The model under review builds one solid part; all positions refer to its coordinate system, in mm. Face numbers are marked on the shaded views. A direction names the side the tool comes from. Coordinates: 2 decimals unless noted, no trailing zeros. Loops run counter-clockwise (first coordinate to the right, second up) from the corner with the lowest first, then second, coordinate; pieces in that order, holes last. Notation, with made-up numbers: M 70,36.25 L 117,36.25 A23 cw 117,52.25 Z; hole C -11,28.25 d7. An arc over 180 degrees is marked long. Write item = value, one per line. Start each with the question number.
Q1. Mouldability with a two-part tool opening along Y and no side actions: class the marked faces 4, 5, 6 and 7 as released by +Y, released by -Y, zero draft, split by the parting line, or undercut.
Q2. Clearance check with flat-ended pins moving along their axes: pin 1 Ø0.8 at (x, z) = (-12.5, 3) entering from -Y; pin 2 Ø1.5 at (y, z) = (7.5, 2.5) entering from -X; pin 3 Ø6 at (x, z) = (-7, 1.5) entering from -Y. State where each tip first meets the part, or that it passes through.
Q3. We need section C-C on z = 9. Give the boundary of the cut face in (x, y), and give its area (3 significant figures).
Q4. For the marked faces 1, 2 and 3, list the 3-axis set-ups (+Z, -Z, +X, -X, +Y, -Y) from which the entire face can be reached by the end or side of a thin tool; tool diameter is ignored.
Q5. We need section B-B on x = 2.5. Give the boundary of the cut face in (y, z), and give its area (3 significant figures).
Q6. We need section D-D on x = -6.5. Give the boundary of the cut face in (y, z).
Q7. Wall thickness on probe 1 along X at (y, z) = (0.25, 1.25); probe 2 along Y at (x, z) = (-1, 9); probe 3 along Y at (x, z) = (4.25, 6.75): over which ranges is each line inside the solid? List them lowest first.
Q8. We need section A-A on y = 1. Give the boundary of the cut face in (x, z), and give its area (3 significant figures).
from build123d import *

# Parameters (mm, degrees)
F1_DEPTH = 10


with BuildPart() as f1:
    # F0 (on Top) → F1 (new body)
    with BuildSketch(Plane.XY):
        with BuildLine():
            ThreePointArc((0, 5.656854), (2.898979, 3.464102), (4, 0))
            ThreePointArc((4, 0), (2.828427, -2.828427), (0, -4))
            ThreePointArc((0, -4), (-3.007566, -2.855084), (-4.492418, 0))
            Line((-4.492418, 0), (-2.992418, 0))
            ThreePointArc((-2.992418, 0), (-4.496209, 1.640499), (-6, 0))
            ThreePointArc((-6, 0), (-4.069705, -3.916951), (0, -5.5))
            ThreePointArc((0, -5.5), (3.889087, -3.889087), (5.5, 0))
            ThreePointArc((5.5, 0), (4.123724, 4.330127), (0.5, 7.071068))
            ThreePointArc((0.5, 7.071068), (-6.330127, 6.123724), (-9.5, 0))
            ThreePointArc((-9.5, 0), (0, -9.5), (9.5, 0))
            ThreePointArc((9.5, 0), (-2, 11.5), (-13.5, 0))
            Line((-13.5, 0), (-12, 0))
            ThreePointArc((-12, 0), (-2, 10), (8, 0))
            ThreePointArc((8, 0), (0, -8), (-8, 0))
            ThreePointArc((-8, 0), (-5.464102, 4.898979), (0, 5.656854))
        make_face()
    extrude(amount=F1_DEPTH)


solid = f1.part
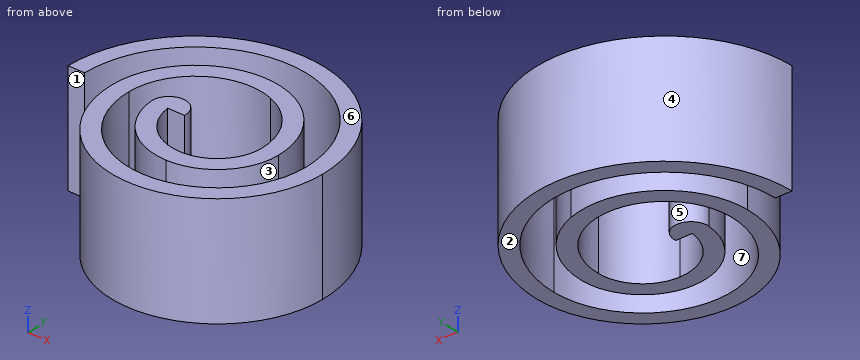
Returned:
q1.face_4 = released by +Y
q1.face_5 = undercut
q1.face_6 = zero draft
q1.face_7 = undercut
q2.pin_1 = 0
q2.pin_2 = -11.31
q2.pin_3 = -8.62
q3.outline = M -13.5,0 L -12,0 A10 cw 8,0 A8 cw -8,0 A6 cw 4,0 A4 cw 0,-4 A4.52 cw -4.49,0 L -2.99,0 A1.51 ccw long -6,0 A6.02 ccw 0,-5.5 A5.5 ccw 5.5,0 A7.5 ccw 0.5,7.07 A7.5 ccw -9.5,0 A9.5 ccw 9.5,0 A11.5 ccw Z
q3.area = 151 mm^2
q4.face_1 = +Z, -Z, -X, -Y
q4.face_2 = -Z, +X, -X, +Y, -Y
q4.face_3 = +Z, -Z
q5.outline = M -9.17,0 L -7.6,0 L -7.6,10 L -9.17,10 Z; M -4.9,0 L -3.12,0 L -3.12,10 L -4.9,10 Z; M 3.97,0 L 6,0 L 6,10 L 3.97,10 Z; M 8.93,0 L 10.58,0 L 10.58,10 L 8.93,10 Z
q5.area = 70.3 mm^2
q6.outline = M -6.93,0 L -4.66,0 L -4.66,10 L -6.93,10 Z; M 3.97,0 L 6,0 L 6,10 L 3.97,10 Z; M 8.93,0 L 10.58,0 L 10.58,10 L 8.93,10 Z
q7.probe_1 = -13.5 to -12, -9.5 to -7.99, -6 to -2.99, 3.99 to 5.5, 8 to 9.5
q7.probe_2 = -9.45 to -7.94, -5.42 to -3.89, 5.92 to 7.43, 9.95 to 11.46
q7.probe_3 = -8.5 to -6.78, -3.49 to 4.15, 7.81 to 9.65
q8.outline = M -13.46,0 L -11.95,0 L -11.95,10 L -13.46,10 Z; M -9.43,0 L -7.92,0 L -7.92,10 L -9.43,10 Z; M -5.73,0 L -3.26,0 L -3.26,10 L -5.73,10 Z; M 3.92,0 L 5.43,0 L 5.43,10 L 3.92,10 Z; M 7.95,0 L 9.46,0 L 9.46,10 L 7.95,10 Z
q8.area = 85.2 mm^2
